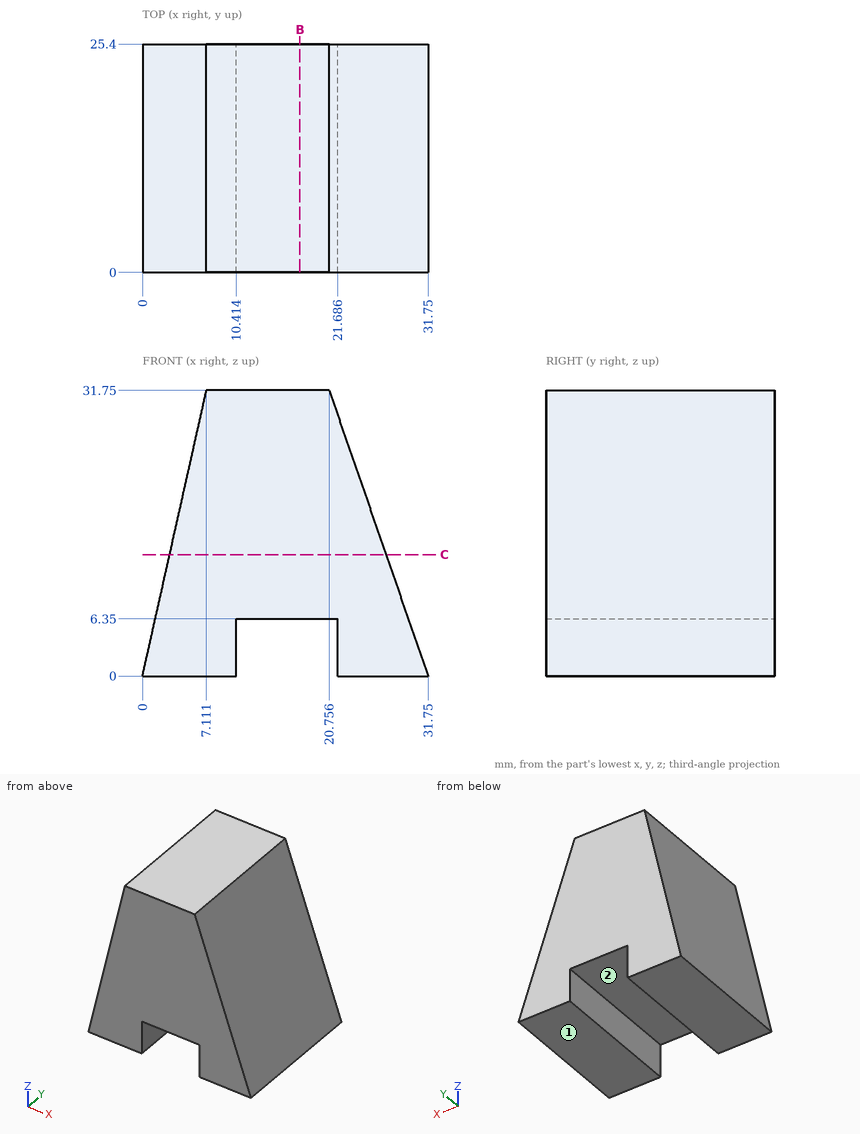
Design review of the part shown in the three views and the two pictorial views. Dimensions are in mm from the part's minimum x, y and z. A direction names the side the tool comes from. Round coordinates to 2 decimals unless told otherwise and drop trailing zeros. Order: outer loops, then holes, each group sorted by start corner. A loop starts at its lowest first (then second) coordinate and runs counter-clockwise, first axis right, second up.
Q1. Machinability: for the marked faces 1 and 2, which of the approach directions +Z, -Z, +X, -X, +Y, -Y give a long, thin tool a straight path to every point of the face, cutting with its end or side? Answer none if there is none.
Findings below:
face 1: -Z, +X, -X, +Y, -Y
face 2: -Z, +Y, -Y
Q2. We need section B-B, the plane x = 17.5. Give the boundary of the cut face in (y, z).
Findings below:
outline: (0, 6.35) - (25.4, 6.35) - (25.4, 31.75) - (0, 31.75) - close
Q3. We need section C-C, the plane z = 13.5. Give the boundary of the cut face in (x, y) (1 decimal), plus the area to 3 significant figures.
Findings below:
outline: (3, 0) - (27.1, 0) - (27.1, 25.4) - (3, 25.4) - close
area: 611 mm2
Q4. Wall thickness on line 1 (Z direction, x = 15, y = 16.5); line 2 (X direction, y = 13.75, z = 18.5) (1 decimal); line 3 (X direction, y = 24, z = 4) (1 decimal): over which ranges is each line inside the solid? List them lowest first.
Findings below:
line 1: z = 6.35 to 31.75
line 2: x = 4.1 to 25.3
line 3: x = 0.9 to 10.4, 21.7 to 30.4
Q5. Insertion check: P1, Ø12, axis at y = 3, z = 18.5, coming from the +X side; P2, Ø5, axis at y = 8, z = 4, coming from the -X side; P3, Ø3, axis at y = 21, z = 6, coming from the -X side. Each pin has a flat end and moves straight along its axis. Give the tip position at first contact, or say it passes through.
Findings below:
P1: stops at x = 27.42
P2: stops at x = 0.34
P3: stops at x = 1.01
